Check sheet for the drawn part. Datum: minimum x, y, z corner. Units: mm. A direction names the side the tool comes from. Coordinates: 2 decimals unless noted, no trailing zeros. Loops run counter-clockwise (first coordinate to the right, second up) from the corner with the lowest first, then second, coordinate; pieces in that order, holes last. Notation, with made-up numbers: (22.5, 88) -> (70.5, 88) arc R29 cw to (70.5, 112) -> close; hole circle Ø8 at (-21, 17). An arc over 180 degrees is marked (long way). Use CSV: the item, a comma, the result in double quotes. Start each with the question number.
1. Set-up check for the marked faces 1 and 2: record each of +Z, -Z, +X, -X, +Y, -Y from which the full face is reachable in a straight line by a thin tool's end or side.
2. Sectioned sample at D-D, the plane z = 11. Record the cut outline in (x, y).
3. Gauge pin test, flat ends, axial feed: pin 1 (1.5 mm diameter, centred on x = 10.5, y = 1.5, fed in from +Z) (1 decimal); pin 2 (1 mm diameter, centred on y = 2, z = 2, fed in from +X) (1 decimal); pin 3 (1.5 mm diameter, centred on x = 4, z = 8, fed in from -Y); pin 4 (1.5 mm diameter, centred on x = 5, y = 1.5, fed in from +Z). Record the tip position at first contact, or that the pin passes through.
4. Thickness scan on L1, parallel to Z at x = 5.75, y = 0.9 (1 decimal); L2, parallel to X at y = 2.3, z = 6 (1 decimal); L3, parallel to Z at x = 8, y = 1.75. Record the ranges inside material, lowest first.
5. Sectioned sample at C-C, the plane y = 1.85. Record the cut outline in (x, z), and give its area (3 significant figures).
6. Sectioned sample at B-B, the plane z = 5.75. Record the cut outline in (x, y).
7. Sectioned sample at A-A, the plane x = 7.25. Record the cut outline in (y, z) (1 decimal).
8. Release check for a two-part mould opening along Z. For the marked faces 3, 4 and 5 record: pulls with the +Z half, pulls with the -Z half, needs draft (parallel to the pull), parting line crosses it, or undercut.
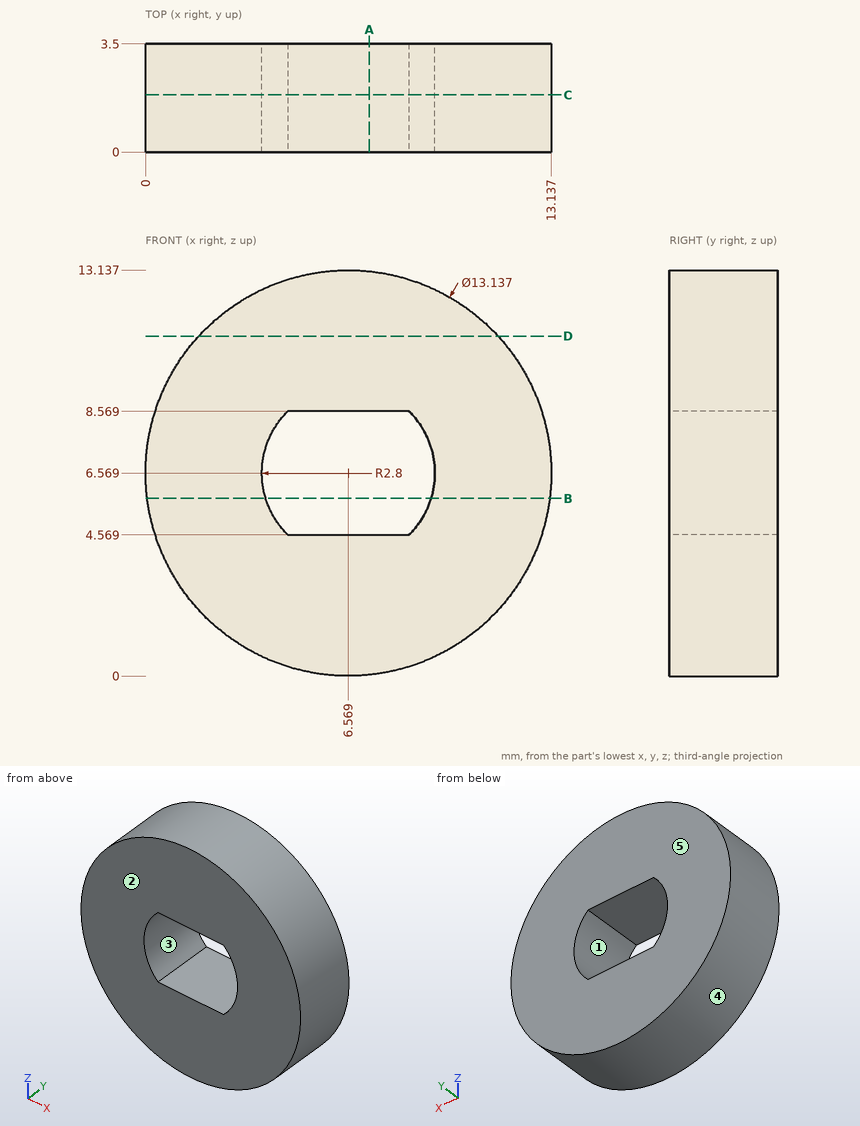
Completed:
1,face 1,"+Y, -Y"
1,face 2,"+Z, -Z, +X, -X, -Y"
2,outline,"(1.72, 0) -> (11.42, 0) -> (11.42, 3.5) -> (1.72, 3.5) -> close"
3,pin 1,"z = 12.3"
3,pin 2,"x = 11.7"
3,pin 3,"y = 0"
3,pin 4,"z = 13.09"
4,L1,"0.1 to 4.6, 8.6 to 13.1"
4,L2,"0 to 3.8, 9.3 to 13.1"
4,L3,"0.16 to 4.57, 8.57 to 12.98"
5,outline,"circle Ø13.14 at (6.57, 6.57); hole (4.61, 4.57) -> (8.53, 4.57) arc R2.8 ccw to (8.53, 8.57) -> (4.61, 8.57) arc R2.8 ccw to start"
5,area,"115 mm²"
6,outline,"(0.05, 0) -> (3.89, 0) -> (3.89, 3.5) -> (0.05, 3.5) -> close; (9.25, 0) -> (13.09, 0) -> (13.09, 3.5) -> (9.25, 3.5) -> close"
7,outline,"(0, 0) -> (3.5, 0) -> (3.5, 4.6) -> (0, 4.6) -> close; (0, 8.6) -> (3.5, 8.6) -> (3.5, 13.1) -> (0, 13.1) -> close"
8,face 3,"undercut"
8,face 4,"parting line crosses it"
8,face 5,"needs draft"
